For this review, take the finished solid that the model builds, in its own axes (mm). Face numbers are marked on the shaded views. A direction names the side the tool comes from. Round coordinates to 2 decimals unless told otherwise and drop trailing zeros. Loops run counter-clockwise (first coordinate to the right, second up) from the corner with the lowest first, then second, coordinate; pieces in that order, holes last.
```python
from build123d import *

# Parameters (mm, degrees)
PROFILE_LASER_PROFILE_3P5_W   = 3.5
PROFILE_LASER_PROFILE_3P5_H   = 3
PROFILE_LASER_PROFILE_3P5_W_2 = 6
PROFILE_LASER_PROFILE_3P5_H_2 = 3.5
PROFILE_LASER_PROFILE_3P5_H_3 = 10
LASER_PROFILE_3P5_DEPTH       = 3.5


with BuildPart() as part:
    # Profile_Laser_profile_3p5 → Laser_profile_3p5 (new body)
    with BuildSketch(Plane.XY):
        Polygon((0, 30.427227289), (8, 18), (4, 18), (12, 7), (10, 7), (14, -7), (10, -7), (14, -20), (10, -20), (14, -33), (4, -33), (4, -49.572772711), (-4, -49.572772711), (-4, -33), (-14, -33), (-10, -20), (-14, -20), (-10, -7), (-14, -7), (-10, 7), (-12, 7), (-4, 18), (-8, 18), align=None)
        with Locations((-7, 3.5)):
            Rectangle(PROFILE_LASER_PROFILE_3P5_W, PROFILE_LASER_PROFILE_3P5_H, mode=Mode.SUBTRACT)
        with Locations((-7, -2.5)):
            Rectangle(PROFILE_LASER_PROFILE_3P5_W, PROFILE_LASER_PROFILE_3P5_H, mode=Mode.SUBTRACT)
        with Locations((-7, -25.5)):
            Rectangle(PROFILE_LASER_PROFILE_3P5_W, PROFILE_LASER_PROFILE_3P5_H, mode=Mode.SUBTRACT)
        with Locations((7, 3.5)):
            Rectangle(PROFILE_LASER_PROFILE_3P5_W, PROFILE_LASER_PROFILE_3P5_H, mode=Mode.SUBTRACT)
        with Locations((7, -2.5)):
            Rectangle(PROFILE_LASER_PROFILE_3P5_W, PROFILE_LASER_PROFILE_3P5_H, mode=Mode.SUBTRACT)
        with Locations((7, -25.5)):
            Rectangle(PROFILE_LASER_PROFILE_3P5_W, PROFILE_LASER_PROFILE_3P5_H, mode=Mode.SUBTRACT)
        with Locations((0, -10.25)):
            Rectangle(PROFILE_LASER_PROFILE_3P5_W_2, PROFILE_LASER_PROFILE_3P5_H_2, mode=Mode.SUBTRACT)
        Rectangle(PROFILE_LASER_PROFILE_3P5_W_2, PROFILE_LASER_PROFILE_3P5_H_3, mode=Mode.SUBTRACT)
    extrude(amount=LASER_PROFILE_3P5_DEPTH)


solid = part.part
```
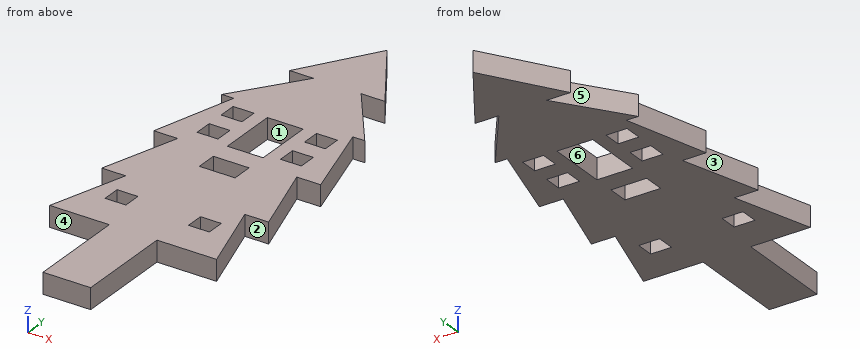
(1) Add section D-D (y = -45). Give the boundary of the cut face in (x, z).
(2) Add section C-C (z = 1.5). Give the number of separate pieces and of enclosed holes in the cut face, plus the area to 3 significant figures.
(3) Add section A-A (x = 2). Give the boundary of the cut face in (y, z).
(4) The part is to be moulded in two halves that separate along X. For the marked faces 1, 2 and 3, say which applies: pulls with the +X half, pulls with the -X half, needs draft (parallel to the pull), parting line crosses it, or undercut.
(5) Insertion check: pin 1 Ø1 at (x, z) = (-6, 1) entering from -Y; pin 2 Ø0.9 at (y, z) = (-3, 1) entering from +X; pin 3 Ø0.9 at (y, z) = (-3, 2) entering from -X; pin 4 Ø6 at (x, y) = (11, 15.5) entering from -Z. Each pin has a flat end and moves straight along its axis. Give the tip position at first contact, or say it passes through.
(6) For L1, parallel to Y at x = 5.5, z = 1.05; L2, parallel to Y at x = -1.75, z = 2.3; L3, parallel to Y at x = 8.5, z = 1.2, list the stretches that pass through material, from the lowest coordinate up.
(7) Add section B-B (y = -10.5). Give the boundary of the cut face in (x, z).
(8) For the marked faces 4, 5 and 6, list the 3-axis set-ups (+Z, -Z, +X, -X, +Y, -Y) from which the entire face can be reached by the end or side of a thin tool; tool diameter is ignored.
Outcome:
1. outline: (-4, 0) - (4, 0) - (4, 3.5) - (-4, 3.5) - close
2. separate pieces: 1
2. enclosed holes: 8
2. area: 1,220 mm2
3. outline: (-49.57, 0) - (-12, 0) - (-12, 3.5) - (-49.57, 3.5) - close; (-8.5, 0) - (-5, 0) - (-5, 3.5) - (-8.5, 3.5) - close; (5, 0) - (27.32, 0) - (27.32, 3.5) - (5, 3.5) - close
4. face 1: undercut
4. face 2: needs draft
4. face 3: pulls with the -X half
5. pin 1: stops at y = -33
5. pin 2: stops at x = 12.99
5. pin 3: stops at x = -12.99
5. pin 4: passes through
6. L1: y = -33 to -27, -24 to -4, -1 to 2, 5 to 15.94, 18 to 21.88
6. L2: y = -49.57 to -12, -8.5 to -5, 5 to 27.71
6. L3: y = -33 to -27, -24 to -4, -1 to 2, 5 to 11.81
7. outline: (-11.08, 0) - (-3, 0) - (-3, 3.5) - (-11.08, 3.5) - close; (3, 0) - (11.08, 0) - (11.08, 3.5) - (3, 3.5) - close
8. face 4: +Z, -Z, -X, -Y
8. face 5: +Z, -Z, -X
8. face 6: +Z, -Z
